```python
from build123d import *

# Parameters (mm, degrees)
SKETCH1_R           = 46.575911122
SKETCH1_R_2         = 1.5875
SKETCH1_R_3         = 1.587499998
BOSS_EXTRUDE1_DEPTH = 3.175


with BuildPart() as part:
    # Sketch1 → Boss-Extrude1 (new body)
    with BuildSketch(Plane(origin=(0, 0, 0), x_dir=(1, 0, 0), z_dir=(0, 1, 0))):
        with Locations(Location((-1e-09, 0, 0), (0, 0, 270))):
            Circle(SKETCH1_R)
        with Locations(Location((24.022660032, -28.55227459, 0), (0, 0, 270))):
            Circle(SKETCH1_R_2, mode=Mode.SUBTRACT)
        with Locations(Location((-24.237339968, -28.55227459, 0), (0, 0, 270))):
            Circle(SKETCH1_R_3, mode=Mode.SUBTRACT)
        with Locations(Location((-21.062339968, 37.48772541, 0), (0, 0, 270))):
            Circle(SKETCH1_R_2, mode=Mode.SUBTRACT)
        with Locations(Location((20.847660032, 37.48772541, 0), (0, 0, 270))):
            Circle(SKETCH1_R_2, mode=Mode.SUBTRACT)
        with BuildLine():
            Line((-1.12253199, -10.1027881), (-17.640592509, -26.62084862))
            ThreePointArc((-17.640592509, -26.62084862), (-18.09333437, -27.940023623), (-17.330191539, -29.107418543))
            ThreePointArc((-17.330191539, -29.107418543), (1.9e-08, -33.875911102), (17.330191572, -29.107418523))
            ThreePointArc((17.330191572, -29.107418523), (18.093334404, -27.940023602), (17.640592543, -26.620848599))
            Line((17.640592543, -26.620848599), (1.12253204, -10.1027881))
            ThreePointArc((1.12253204, -10.1027881), (2.5e-08, -9.637820115), (-1.12253199, -10.1027881))
        make_face(mode=Mode.SUBTRACT)
        with BuildLine():
            Line((-10.102788112, 1.122532053), (-26.6208486, 17.640592539))
            ThreePointArc((-26.6208486, 17.640592539), (-27.940023602, 18.093334401), (-29.107418522, 17.330191571))
            ThreePointArc((-29.107418522, 17.330191571), (-33.875911101, 2.9e-08), (-29.107418553, -17.330191521))
            ThreePointArc((-29.107418553, -17.330191521), (-27.940023632, -18.093334356), (-26.620848627, -17.640592494))
            Line((-26.620848627, -17.640592494), (-10.102788113, -1.122531976))
            ThreePointArc((-10.102788113, -1.122531976), (-9.637820128, 3.8e-08), (-10.102788112, 1.122532053))
        make_face(mode=Mode.SUBTRACT)
        with BuildLine():
            Line((1.122532046, 10.102788181), (17.640592494, 26.620848628))
            ThreePointArc((17.640592494, 26.620848628), (18.093334353, 27.940023632), (17.33019152, 29.107418551))
            ThreePointArc((17.33019152, 29.107418551), (2.4e-08, 33.8759111), (-17.33019148, 29.107418577))
            ThreePointArc((-17.33019148, 29.107418577), (-18.093334314, 27.940023657), (-17.640592454, 26.620848652))
            Line((-17.640592454, 26.620848652), (-1.122531984, 10.102788181))
            ThreePointArc((-1.122531984, 10.102788181), (3.1e-08, 9.637820197), (1.122532046, 10.102788181))
        make_face(mode=Mode.SUBTRACT)
        with BuildLine():
            Line((26.620848619, 17.64059251), (10.102788169, 1.12253206))
            ThreePointArc((10.102788169, 1.12253206), (9.637820183, 4.4e-08), (10.102788168, -1.122531972))
            Line((10.102788168, -1.122531972), (26.620848653, -17.640592453))
            ThreePointArc((26.620848653, -17.640592453), (27.940023657, -18.093334314), (29.107418578, -17.33019148))
            ThreePointArc((29.107418578, -17.33019148), (33.875911102, 3.4e-08), (29.107418542, 17.330191539))
            ThreePointArc((29.107418542, 17.330191539), (27.940023622, 18.09333437), (26.620848619, 17.64059251))
        make_face(mode=Mode.SUBTRACT)
        Polygon((-19.083044242, -16.837980228), (-16.837980211, -19.083044257), (-3.367596019, -5.612660086), (-5.61266005, -3.367596056), align=None, mode=Mode.SUBTRACT)
        Polygon((16.837980228, -19.083044242), (19.083044257, -16.837980211), (5.612660086, -3.367596019), (3.367596056, -5.61266005), align=None, mode=Mode.SUBTRACT)
        Polygon((19.083044242, 16.837980228), (16.837980211, 19.083044257), (3.367596019, 5.612660086), (5.61266005, 3.367596056), align=None, mode=Mode.SUBTRACT)
        Polygon((-16.837980228, 19.083044242), (-19.083044257, 16.837980211), (-5.612660086, 3.367596019), (-3.367596056, 5.61266005), align=None, mode=Mode.SUBTRACT)
    extrude(amount=BOSS_EXTRUDE1_DEPTH)


solid = part.part
```
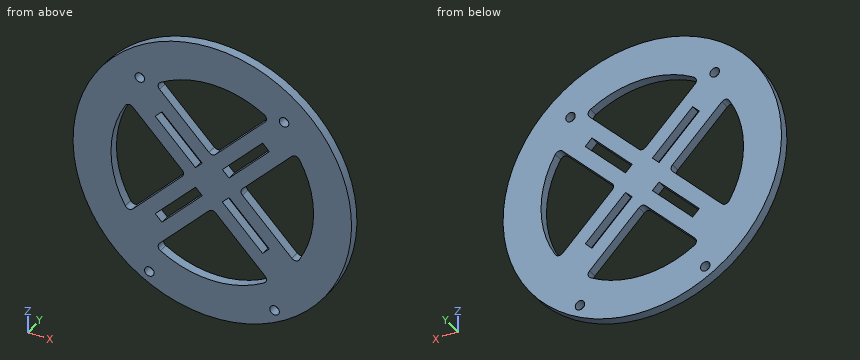
Geometry check sheet. Reference: the model listing, model coordinates, mm. Coordinates: 2 decimals unless noted, no trailing zeros. Order: outer loops, then holes, each group sorted by start corner. A loop starts at its lowest first (then second) coordinate and runs counter-clockwise, first axis right, second up. Notation, with made-up numbers: M -9,-9.75 L 40,-9.75 A24 cw 40,14.25 Z; hole C -34,-35.75 d2. An arc over 180 degrees is marked long. One line per question, with ' | ' between items. Start each with the question number.
Item 1: Material ranges on L1, parallel to Z at x = 2.5, y = 0.7; L2, parallel to Z at x = 15, y = 1.25; L3, parallel to X at y = 0.5, z = 16, recorded low to high. Write a range as [from, to].
Item 2: Gauge pin test, flat end, axial feed: pin 1 (1 mm diameter, centred on y = 0.5, z = -33.5, fed in from -X). Record the tip position at first contact, or that the pin passes through.
Item 3: Cross-section at A-A on x = 0. Enter the section's corners in (y, z) (3 decimals).
Item 4: Cross-section at D-D on x = -12.5. Enter the section's corners in (y, z) (3 decimals).
Item 5: Cross-section at B-B on z = -28. Enter the section's corners in (x, y) (3 decimals), then the cut area to 3 significant figures.
Item 6: Cross-section at C-C on z = 0. Enter the section's corners in (x, y) (3 decimals), then the cut area to 3 significant figures.
Findings:
1) L1: z = [-46.51, -33.78], [-11.48, 11.48], [33.78, 46.51] | L2: z = [-44.09, -30.37], [-23.98, -17.25], [-12.75, -6.02], [6.02, 12.75], [17.25, 23.98], [30.37, 44.09] | L3: x = [-43.74, -29.86], [-24.98, -18.25], [-13.75, -7.02], [7.02, 13.75], [18.25, 24.98], [29.86, 43.74]
2) pin 1: stops at x = -32.87
3) outline: M 0,-46.576 L 3.175,-46.576 L 3.175,-33.876 L 0,-33.876 Z; M 0,-9.638 L 3.175,-9.638 L 3.175,9.638 L 0,9.638 Z; M 0,33.876 L 3.175,33.876 L 3.175,46.576 L 0,46.576 Z
4) outline: M 0,-44.867 L 3.175,-44.867 L 3.175,-31.485 L 0,-31.485 Z; M 0,-21.48 L 3.175,-21.48 L 3.175,-14.745 L 0,-14.745 Z; M 0,-10.255 L 3.175,-10.255 L 3.175,-3.52 L 0,-3.52 Z; M 0,3.52 L 3.175,3.52 L 3.175,10.255 L 0,10.255 Z; M 0,14.745 L 3.175,14.745 L 3.175,21.48 L 0,21.48 Z; M 0,31.485 L 3.175,31.485 L 3.175,44.867 L 0,44.867 Z
5) outline: M -37.22,0 L -18.085,0 L -18.085,3.175 L -37.22,3.175 Z; M 18.085,0 L 37.22,0 L 37.22,3.175 L 18.085,3.175 Z | area: 122 mm²
6) outline: M -46.576,0 L -33.876,0 L -33.876,3.175 L -46.576,3.175 Z; M -9.638,0 L 9.638,0 L 9.638,3.175 L -9.638,3.175 Z; M 33.876,0 L 46.576,0 L 46.576,3.175 L 33.876,3.175 Z | area: 142 mm²
